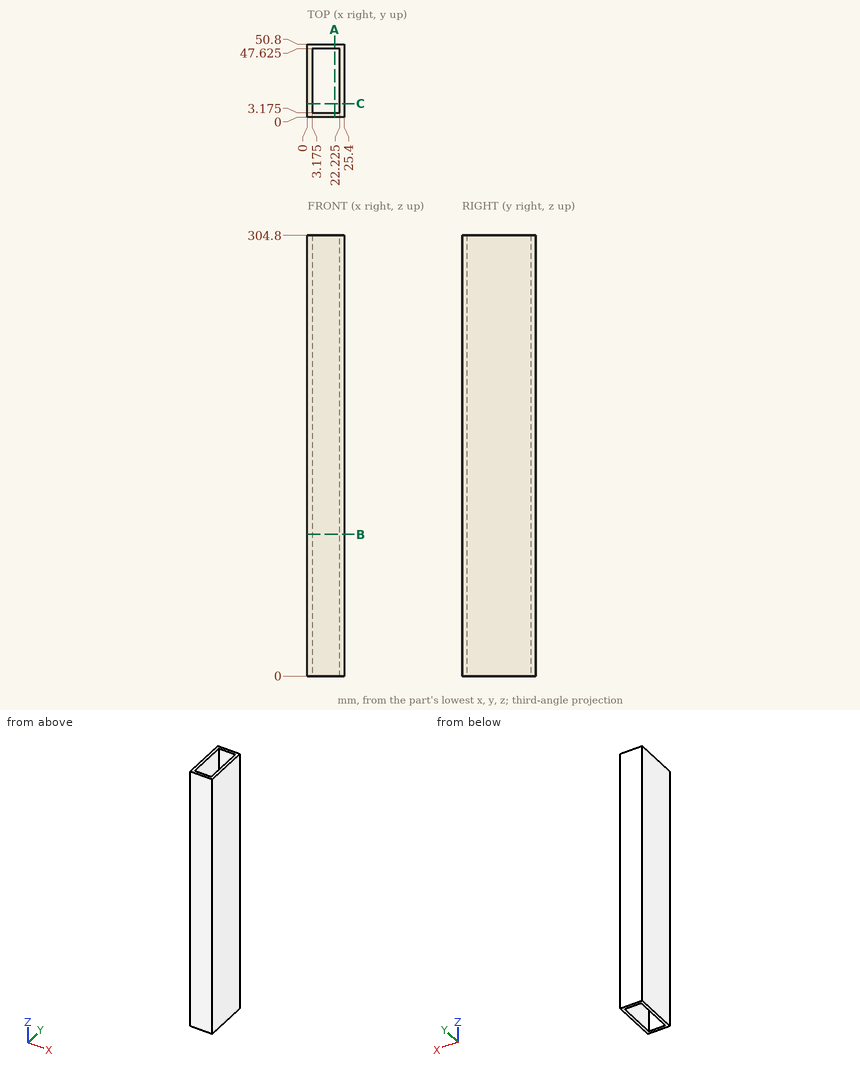
Answer from the drawing. Dimensions are ordinates in mm from the lowest x, y and z of the part. Coordinates: 2 decimals unless noted, no trailing zeros. Order: outer loops, then holes, each group sorted by start corner. A loop starts at its lowest first (then second) coordinate and runs counter-clockwise, first axis right, second up. Notation, with made-up numbers: M 44,36.5 L 48,36.5 A13 ccw 48,45.5 Z; hole C 52.25,75 d10. An arc over 180 degrees is marked long. Put each result on its own line as item: value. Start each with the question number.
Item 1: Consider probe 1 along X at (y, z) = (45, 141.5) (3 decimals); probe 2 along Y at (x, z) = (14.5, 275) (3 decimals). Determine where each line is inside the solid, lowest interval first. Write a range as [from, to].
Item 2: Section C-C, the plane y = 9.5 is taken. Determine the outline of the cut face in (x, z) (3 decimals), plus the area to 3 significant figures.
Item 3: Section A-A, the plane x = 18.75 is taken. Determine the outline of the cut face in (y, z) (3 decimals).
Item 4: Section B-B, the plane z = 98 is taken. Determine the outline of the cut face in (x, y) (3 decimals).
Computed:
1. probe 1: x = [0, 3.175], [22.225, 25.4]
1. probe 2: y = [0, 3.175], [47.625, 50.8]
2. outline: M 0,0 L 3.175,0 L 3.175,304.8 L 0,304.8 Z; M 22.225,0 L 25.4,0 L 25.4,304.8 L 22.225,304.8 Z
2. area: 1,940 mm2
3. outline: M 0,0 L 3.175,0 L 3.175,304.8 L 0,304.8 Z; M 47.625,0 L 50.8,0 L 50.8,304.8 L 47.625,304.8 Z
4. outline: M 0,0 L 25.4,0 L 25.4,50.8 L 0,50.8 Z; hole M 3.175,3.175 L 22.225,3.175 L 22.225,47.625 L 3.175,47.625 Z
